Here's how the part is built. I have some questions about the finished solid (model axes, mm). Face numbers are marked on the shaded views. A direction names the side the tool comes from. Round coordinates to 2 decimals unless told otherwise and drop trailing zeros. Write each loop counter-clockwise with the first axis right and the second up, starting at its lowest first coordinate (ties: lowest second). Pieces come first, ordered by that corner, then holes. Notation, with made-up numbers: (6.25, 0.5) -> (52.25, 0.5) arc R16 ccw to (52.25, 26.5) -> close; hole circle Ø9 at (58.25, -33.5). An arc over 180 degrees is marked (long way). Put each result on its own line as item: value. Start each with the question number.
1. I need wall thicknesses on probe 1 along Y at (x, z) = (-8, 2.5); probe 2 along Y at (x, z) = (-24, 4); probe 3 along X at (y, z) = (8, 3.5). Which ranges of each line are inside material? Lowest first, please. Write a range as from..to.
2. Which directions (+Z, -Z, +X, -X, +Y, -Y) give clear straight access to the entire face, cutting with the end or side of a thin tool? Please do the marked faces 1 and 2.
3. Suppose I cut it at A-A (y = -5.1). Please give me the cut outline in (x, z), then the cut area to 3 significant figures.
4. Suppose I cut it at B-B (z = 1.75). Please give me the cut outline in (x, y).
5. Suppose I cut it at C-C (z = 7). Please give me the cut outline in (x, y).
6. For pin 1 (6 mm diameter, centred on x = 0.5, y = -0.5, fed in from -Z); pin 2 (5 mm diameter, centred on x = -0.5, y = 44.5, fed in from -Z); pin 3 (1 mm diameter, centred on x = -21.5, z = 1.5, fed in from +Y); pin 4 (2.5 mm diameter, centred on y = 40, z = 3.5, fed in from -X), each with a flat end and sliding along its axis, tell me the tip position at first contact or that it passes through.
7. Suppose I cut it at D-D (y = -30). Please give me the cut outline in (x, z), then the cut area to 3 significant figures.
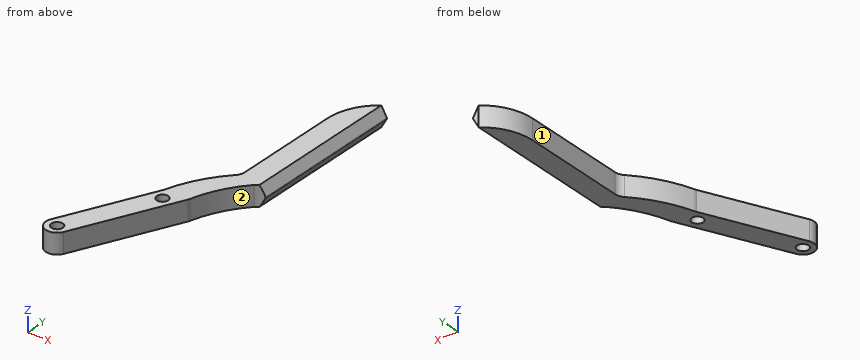
```python
from build123d import *

# Parameters (mm, degrees)
SKETCH1_R           = 2.55
BOSS_EXTRUDE1_DEPTH = 9
SKETCH2_W           = 1.5
SKETCH2_H           = 71.301363943
CUT_EXTRUDE1_DEPTH  = 10
BOSS_EXTRUDE2_DEPTH = 70.2819
FILLET1_R           = 0.5
FILLET2_R           = 5


with BuildPart() as part:
    # Sketch1 → Boss-Extrude1 (new body)
    with BuildSketch(Plane.XY):
        with BuildLine():
            Line((-11.03377919, 0), (-30.17656458, -41.051835747))
            ThreePointArc((-30.17656458, -41.051835747), (-27.758116953, -47.696465991), (-21.113486709, -45.278018364))
            Line((-21.113486709, -45.278018364), (0, 0))
            ThreePointArc((0, 0), (5.686222606, 13.627582704), (15.104941349, 25))
            Line((15.104941349, 25), (15.104941349, 94.9))
            ThreePointArc((15.104941349, 94.9), (7.014188798, 86.377107313), (4.071162159, 75))
            Line((4.071162159, 75), (4.071162159, 25))
            ThreePointArc((4.071162159, 25), (-5.128820408, 13.495422821), (-11.03377919, 0))
        make_face()
        with Locations((-25.645025645, -43.164927056)):
            Circle(SKETCH1_R, mode=Mode.SUBTRACT)
        with Locations((-7.895058651, -5.1)):
            Circle(SKETCH1_R, mode=Mode.SUBTRACT)
    extrude(amount=BOSS_EXTRUDE1_DEPTH)

    # Sketch2 → Cut-Extrude1 (cut, through all)
    with BuildSketch(Plane.XY.offset(9)):
        with Locations((14.354941349, 59.249318028)):
            Rectangle(SKETCH2_W, SKETCH2_H)
    extrude(amount=-CUT_EXTRUDE1_DEPTH, mode=Mode.SUBTRACT)

    # Sketch4 → Boss-Extrude2 (add)
    with BuildSketch(Plane(origin=(0, 93.880535659, 0), x_dir=(0, 0, -1), z_dir=(0, -1, 0))):
        Polygon((0, 13.604941349), (-4.5, 16.20301756), (-9, 13.604941349), align=None)
    extrude(amount=BOSS_EXTRUDE2_DEPTH)

    # Fillet1
    fillet1_edges = [part.edges().sort_by_distance(p)[0] for p in [
        (16.20301756, 58.739585659, 4.5),
    ]]
    fillet(fillet1_edges, radius=FILLET1_R)

    # Fillet2
    fillet2_edges = [part.edges().sort_by_distance(p)[0] for p in [
        (0, 0, 4.5),
        (-11.03377919, 0, 4.5),
        (4.071162159, 25, 4.5),
        (13.604941349, 23.598636057, 4.5),
    ]]
    fillet(fillet2_edges, radius=FILLET2_R)


solid = part.part
```
Verdict:
1. probe 1: y = -17.16..-7.65, -2.55..8.1
1. probe 2: y = -47.89..-45.11, -41.22..-27.81
1. probe 3: x = -8.05..2.76
2. face 1: +Z, -Z, -X, +Y
2. face 2: +Z, -Z, +X, -Y
3. outline: (-13.41, 0) -> (-10.45, 0) -> (-10.45, 9) -> (-13.41, 9) -> close; (-5.35, 0) -> (-2.38, 0) -> (-2.38, 9) -> (-5.35, 9) -> close
3. area: 53.4 mm^2
4. outline: (-30.18, -41.05) arc R5 ccw to (-21.11, -45.28) -> (-0.2, -0.42) arc R5 ccw to (0.11, 0.43) arc R50 cw to (12.06, 22.02) arc R5 cw to (14.62, 23.48) -> (14.62, 93.88) -> (13.6, 93.88) arc R23.46 ccw to (4.07, 75) -> (4.07, 27.08) arc R5 cw to (2.66, 23.6) arc R56.37 ccw to (-10.93, 0.35) arc R5 cw to (-11.19, -0.34) -> close; hole circle Ø5.1 at (-25.65, -43.16); hole circle Ø5.1 at (-7.9, -5.1)
5. outline: (-30.18, -41.05) arc R5 ccw to (-21.11, -45.28) -> (-0.2, -0.42) arc R5 ccw to (0.11, 0.43) arc R50 cw to (12.06, 22.02) arc R5 cw to (14.76, 23.51) -> (14.76, 93.88) -> (13.6, 93.88) arc R23.46 ccw to (4.07, 75) -> (4.07, 27.08) arc R5 cw to (2.66, 23.6) arc R56.37 ccw to (-10.93, 0.35) arc R5 cw to (-11.19, -0.34) -> close; hole circle Ø5.1 at (-25.65, -43.16); hole circle Ø5.1 at (-7.9, -5.1)
6. pin 1: stops at z = 0
6. pin 2: passes through
6. pin 3: stops at y = -21.37
6. pin 4: stops at x = 4.07
7. outline: (-25.02, 0) -> (-13.99, 0) -> (-13.99, 9) -> (-25.02, 9) -> close
7. area: 99.3 mm^2
